from build123d import *

# Parameters (mm, degrees)
SKETCH_1_W          = 88.39
SKETCH_1_H          = 150
EXTRUDE_1_DEPTH     = 5
SKETCH_2_R          = 7.5
EXTRUDE_2_DEPTH     = 15
HOLE_WIZARD_1_D     = 8
EXTRUDE_3_DEPTH     = 15
SKETCH_8_R          = 4
CUT_EXTRUDE_1_DEPTH = 166.891205614


with BuildPart() as part:
    # 스케치1 → 보스-돌출1 (new body)
    with BuildSketch(Plane.XY):
        with Locations((44.195, 75)):
            Rectangle(SKETCH_1_W, SKETCH_1_H)
    extrude(amount=EXTRUDE_1_DEPTH)

    # 스케치2 → 보스-돌출2 (add)
    with BuildSketch(Plane(origin=(0, 150, 0), x_dir=(1, 0, 0), z_dir=(0, 1, 0))):
        with Locations((88.39, -2.5)):
            Circle(SKETCH_2_R)
        with Locations((0, -2.5)):
            Circle(SKETCH_2_R)
    extrude(amount=-EXTRUDE_2_DEPTH)

    # 구멍1 (through all)
    with Locations(Plane(origin=(0, 150, 0), x_dir=(1, 0, 0), z_dir=(0, 1, 0))):
        with Locations((0, -2.5), (88.39, -2.5)):
            Hole(HOLE_WIZARD_1_D / 2)

    # 스케치7 → 보스-돌출3 (add)
    with BuildSketch(Plane.XZ):
        with BuildLine():
            Line((81.318932188, 0), (85.267501001, 0))
            ThreePointArc((85.267501001, 0), (84.39, 2.5), (85.267501001, 5))
            Line((85.267501001, 5), (81.318932188, 5))
            ThreePointArc((81.318932188, 5), (95.89, 2.5), (81.318932188, 0))
        make_face()
        with BuildLine():
            Line((3.122498999, 5), (7.071067812, 5))
            ThreePointArc((7.071067812, 5), (-7.5, 2.5), (7.071067812, 0))
            Line((7.071067812, 0), (3.122498999, 0))
            ThreePointArc((3.122498999, 0), (4, 2.5), (3.122498999, 5))
        make_face()
    extrude(amount=-EXTRUDE_3_DEPTH)

    # 스케치8 → 컷-돌출1 (cut, through all)
    with BuildSketch(Plane(origin=(0, 15, 0), x_dir=(1, 0, 0), z_dir=(0, 1, 0))):
        with Locations(Location((0, -2.5, 0), (0, 0, 270))):
            Circle(SKETCH_8_R)
        with Locations(Location((88.39, -2.5, 0), (0, 0, 270))):
            Circle(SKETCH_8_R)
    extrude(amount=-CUT_EXTRUDE_1_DEPTH, mode=Mode.SUBTRACT)


solid = part.part
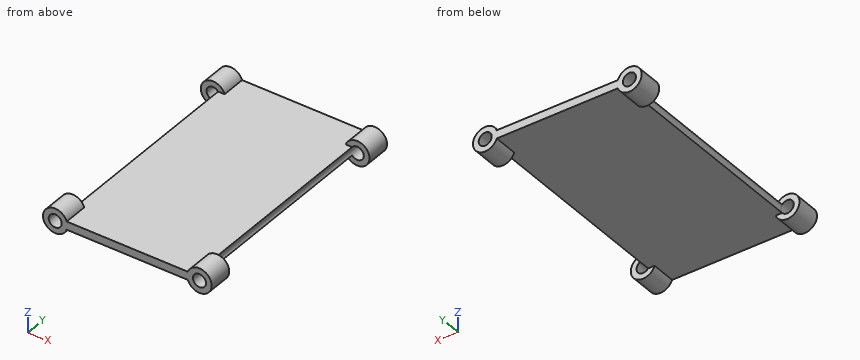
Can you work these out from the model? Positions are in its coordinate system, mm. Round coordinates to 2 decimals unless told otherwise and drop trailing zeros. Order: outer loops, then holes, each group sorted by start corner. A loop starts at its lowest first (then second) coordinate and runs counter-clockwise, first axis right, second up. Notation, with made-up numbers: (77.25, -38.5) - (97.25, -38.5) arc R29 ccw to (97.25, -14.5) - close; hole circle Ø1 at (-33.5, 47.25). An arc over 180 degrees is marked (long way). Answer in a Markdown table with one row per item.
(1) Suppose I cut it at C-C, the plane y = 114. Please give me the cut outline in (x, z).
From the geometry:
| item | result |
|---|---|
| outline | (3.12, 0) - (85.27, 0) arc R4 cw to (85.27, 5) - (3.12, 5) arc R4 cw to start |
(2) For P1, Ø5, axis at x = 69, y = 90.5, coming from the -Z side; P2, Ø9, axis at x = 0, z = 2.5, coming from the -Y side; P3, Ø1.5, axis at y = 36, z = 4.5, coming from the +X side; P4, Ø1, axis at x = 4.5, y = 124.5, coming from the +Z side, each with a flat end and sliding along its axis, tell me the tip position at first contact or that it passes through.
From the geometry:
| item | result |
|---|---|
| P1 | stops at z = 0 |
| P2 | stops at y = 0 |
| P3 | stops at x = 85.27 |
| P4 | stops at z = 5 |
(3) Please list where these lines run through material, in increasing order: L1, parallel to X at y = 3, z = 2.5; L2, parallel to Z at x = 0, y = 5.75; L3, parallel to Z at x = 80.5, y = 64.5. Write a range as from..to.
From the geometry:
| item | result |
|---|---|
| L1 | x = -7.5..-4, 4..84.39, 92.39..95.89 |
| L2 | z = -5..-1.5, 6.5..10 |
| L3 | z = 0..5 |
(4) Suppose I cut it at B-B, the plane z = 2.5. Please give me the cut outline in (x, y), plus the area to 3 significant figures.
From the geometry:
| item | result |
|---|---|
| outline | (-7.5, 0) - (-4, 0) - (-4, 15) - (-7.5, 15) - close; (-7.5, 135) - (-4, 135) - (-4, 150) - (-7.5, 150) - close; (4, 0) - (84.39, 0) - (84.39, 150) - (4, 150) - close; (92.39, 0) - (95.89, 0) - (95.89, 15) - (92.39, 15) - close; (92.39, 135) - (95.89, 135) - (95.89, 150) - (92.39, 150) - close |
| area | 12,300 mm2 |
(5) Suppose I cut it at A-A, the plane x = 0. Please give me the cut outline in (y, z), plus the area to 3 significant figures.
From the geometry:
| item | result |
|---|---|
| outline | (0, -5) - (15, -5) - (15, -1.5) - (0, -1.5) - close; (0, 6.5) - (15, 6.5) - (15, 10) - (0, 10) - close; (135, -5) - (150, -5) - (150, -1.5) - (135, -1.5) - close; (135, 6.5) - (150, 6.5) - (150, 10) - (135, 10) - close |
| area | 210 mm2 |
(6) Suppose I cut it at D-D, the plane x = 48. Please give me the cut outline in (y, z), plus the area to 3 significant figures.
From the geometry:
| item | result |
|---|---|
| outline | (0, 0) - (150, 0) - (150, 5) - (0, 5) - close |
| area | 750 mm2 |
